Geometry check sheet. Reference: the model listing, model coordinates, mm. Give positions to 0.01 mm unless a question says otherwise; leave off trailing zeros. Write each loop counter-clockwise with the first axis right and the second up, starting at its lowest first coordinate (ties: lowest second). Pieces come first, ordered by that corner, then holes. Notation, with made-up numbers: (53, 36.5) -> (109, 36.5) arc R29 cw to (109, 59.5) -> close; hole circle Ø1 at (4, 60). An arc over 180 degrees is marked (long way). One line per item, written item: value.
from build123d import *

# Parameters (mm, degrees)
SKETCH1_W           = 16
SKETCH1_H           = 15
BOSS_EXTRUDE1_DEPTH = 3
CUT_EXTRUDE1_START  = -4
SKETCH2_R           = 2.4
CUT_EXTRUDE1_DEPTH  = 5


with BuildPart() as part:
    # Sketch1 → Boss-Extrude1 (new body)
    with BuildSketch(Plane(origin=(0, 0, 0), x_dir=(1, 0, 0), z_dir=(0, 1, 0))):
        Rectangle(SKETCH1_W, SKETCH1_H)
    extrude(amount=BOSS_EXTRUDE1_DEPTH)

    # Sketch2 → Cut-Extrude1 (cut)
    with BuildSketch(Plane(origin=(0, 3, 0), x_dir=(1, 0, 0), z_dir=(0, 1, 0)).offset(CUT_EXTRUDE1_START)):
        with Locations((-3.75, 0)):
            Circle(SKETCH2_R)
    cut_extrude1 = extrude(amount=CUT_EXTRUDE1_DEPTH, mode=Mode.SUBTRACT)

    # Mirror1: Cut-Extrude1 across plane
    add(cut_extrude1.mirror(Plane(origin=(0, 0, 0), x_dir=(0, 0, 1), z_dir=(1, 0, 0))), mode=Mode.SUBTRACT)


solid = part.part
1) Scan lines: probe 1 along Z at (x, y) = (-3.75, 2.05); probe 2 along X at (y, z) = (2.15, -1); probe 3 along X at (y, z) = (2.8, 1.5). Record each from-to range of solid material in increasing order.
Verdict:
probe 1: -7.5 to -2.4, 2.4 to 7.5
probe 2: -8 to -5.93, -1.57 to 1.57, 5.93 to 8
probe 3: -8 to -5.62, -1.88 to 1.88, 5.62 to 8
2) Sectioned sample at B-B on z = 0. Record the cut outline in (x, y).
Verdict:
outline: (-8, 0) -> (-6.15, 0) -> (-6.15, 3) -> (-8, 3) -> close; (-1.35, 0) -> (1.35, 0) -> (1.35, 3) -> (-1.35, 3) -> close; (6.15, 0) -> (8, 0) -> (8, 3) -> (6.15, 3) -> close
3) Mould release check, pull along Z, two halves, no side actions. Record for faces 1 (the cylindrical face through (1.46, 1.48, -0.72)), 2 (the flat face through (0, 1, -7.5)), 3 (the flat face through (8, 1, 0)): released by +Z, released by -Z, zero draft, split by the parting line, or undercut.
Verdict:
face 1: undercut
face 2: released by -Z
face 3: zero draft
4) Sectioned sample at C-C on y = 2.3. Record the cut outline in (x, z), plus the area to 3 significant figures.
Verdict:
outline: (-8, -7.5) -> (8, -7.5) -> (8, 7.5) -> (-8, 7.5) -> close; hole circle Ø4.8 at (-3.75, 0); hole circle Ø4.8 at (3.75, 0)
area: 204 mm^2
5) Sectioned sample at D-D on z = 2. Record the cut outline in (x, y), plus the area to 3 significant figures.
Verdict:
outline: (-8, 0) -> (-5.08, 0) -> (-5.08, 3) -> (-8, 3) -> close; (-2.42, 0) -> (2.42, 0) -> (2.42, 3) -> (-2.42, 3) -> close; (5.08, 0) -> (8, 0) -> (8, 3) -> (5.08, 3) -> close
area: 32.1 mm^2
6) Sectioned sample at A-A on x = -3.75. Record the cut outline in (y, z), plus the area to 3 significant figures.
Verdict:
outline: (0, -7.5) -> (3, -7.5) -> (3, -2.4) -> (0, -2.4) -> close; (0, 2.4) -> (3, 2.4) -> (3, 7.5) -> (0, 7.5) -> close
area: 30.6 mm^2
